Could you check a few things on this model? Use its own coordinates, in mm. Face numbers are marked on the shaded views. A direction names the side the tool comes from. Give positions to 0.01 mm unless a question says otherwise; leave off trailing zeros. Loops run counter-clockwise (first coordinate to the right, second up) from the corner with the lowest first, then second, coordinate; pieces in that order, holes last. Notation, with made-up numbers: M 57.5,-27.75 L 90.5,-27.75 A16 ccw 90.5,-5.75 Z; hole C 14.25,-24.5 d4. An arc over 180 degrees is marked long. Answer in a Markdown table with one row per item. Add a question column.
```python
from build123d import *

# Parameters (mm, degrees)
RESSALTO_EXTRUS_O1_DEPTH   = 15
CORTE_EXTRUS_O1_DEPTH      = 59.873508474
CORTE_EXTRUS_O1_DEPTH_BACK = 59.873508474
ESBO_O3_R                  = 5.5
CORTE_EXTRUS_O2_DEPTH      = 2
CORTE_EXTRUS_O2_DEPTH_BACK = 2
ESBO_O4_R                  = 11.5
ESBO_O6_R                  = 1.85
CORTE_EXTRUS_O4_DEPTH      = 64.251561246
CHANFRO1_SIZE              = 1.5


with BuildPart() as part:
    # Esboço1 → Ressalto-extrusão1 (new body)
    with BuildSketch(Plane(origin=(0, 0, 0), x_dir=(1, 0, 0), z_dir=(0, 1, 0))):
        with BuildLine():
            Line((3, 50), (3, 3))
            ThreePointArc((3, 3), (2.121320344, 0.878679656), (0, 0))
            Line((0, 0), (25.4, 0))
            ThreePointArc((25.4, 0), (23.278679656, 0.878679656), (22.4, 3))
            Line((22.4, 3), (22.4, 50))
            ThreePointArc((22.4, 50), (23.864466094, 53.535533906), (27.4, 55))
            Line((27.4, 55), (-2, 55))
            ThreePointArc((-2, 55), (1.535533906, 53.535533906), (3, 50))
        make_face()
    extrude(amount=RESSALTO_EXTRUS_O1_DEPTH)

    # Esboço3 → Corte-extrusão1 (cut, two sides: drawn at the far end of the back side and taken through both)
    with BuildSketch(Plane(origin=(12.7, 0, 0), x_dir=(0, 0, -1), z_dir=(1, 0, 0)).offset(-CORTE_EXTRUS_O1_DEPTH_BACK)):
        with Locations((26.5, 0)):
            Circle(ESBO_O3_R)
    extrude(amount=CORTE_EXTRUS_O1_DEPTH + CORTE_EXTRUS_O1_DEPTH_BACK, mode=Mode.SUBTRACT)

    # Esboço4 → Corte-extrusão2 (cut, two sides: drawn at the far end of the back side and taken through both)
    with BuildSketch(Plane(origin=(12.7, 0, 0), x_dir=(0, 0, -1), z_dir=(1, 0, 0)).offset(-CORTE_EXTRUS_O2_DEPTH_BACK)):
        with Locations((26.5, 0)):
            Circle(ESBO_O4_R)
    extrude(amount=CORTE_EXTRUS_O2_DEPTH + CORTE_EXTRUS_O2_DEPTH_BACK, mode=Mode.SUBTRACT)

    # Esboço6 → Corte-extrusão4 (cut, through all)
    with BuildSketch(Plane.XZ):
        with Locations(Location((16.4, -10.4, 0), (0, 0, 270))):
            Circle(ESBO_O6_R)
        with Locations(Location((9, -47, 0), (0, 0, 270))):
            Circle(ESBO_O6_R)
    extrude(amount=-CORTE_EXTRUS_O4_DEPTH, mode=Mode.SUBTRACT)

    # Chanfro1
    chanfro1_edges = [part.edges().sort_by_distance(p)[0] for p in [
        (16.4, 15, -8.55),
        (9, 15, -45.15),
    ]]
    chamfer(chanfro1_edges, length=CHANFRO1_SIZE)


solid = part.part
```
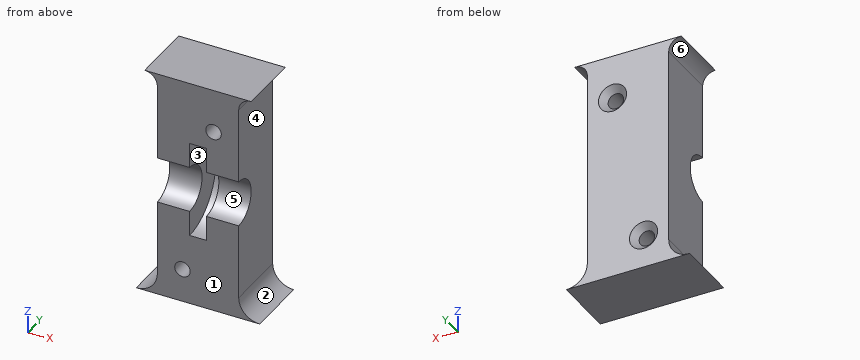
Item 1: If we mould it in two halves opening along X, with no side actions, what happens to the marked faces 1, 2 and 3? For each: +X half, -X half, draft (parallel to the pull), parting line (faces both ways), or undercut.
Item 2: For P1, Ø3.5, axis at y = 4.5, z = -26.5, coming from the -X side; P2, Ø3, axis at y = 4, z = -13, coming from the +X side, each with a flat end and sliding along its axis, tell me the tip position at first contact or that it passes through.
Item 3: Suppose I cut it at C-C (x = 16.4). List the corners of the cut face in (y, z) for me.
Item 4: Suppose I cut it at B-B (z = -10.4). List the corners of the cut face in (x, y) for me, then the cut area to 3 significant figures.
Item 5: Suppose I cut it at A-A (y = 4.5). List the corners of the cut face in (x, z) for me.
Item 6: Suppose I cut it at D-D (y = 12.5). List the corners of the cut face in (x, z) for me, then the cut area to 3 significant figures.
Item 7: For the marked faces 4, 5 and 6, which set-ups out of +Z, -Z, +X, -X, +Y, -Y let a thin tool reach every point of the face, with its end or its side?
Item 8: I need wall thicknesses on L1, parallel to X at y = 9.75, z = -31; L2, parallel to X at y = 10, z = -10.4; L3, parallel to Y at x = 8, z = -26.5. Which ranges of each line are inside material? Lowest first, please.
Values found:
| question | item | result |
|---|---|---|
| 1 | face 1 | draft |
| 1 | face 2 | +X half |
| 1 | face 3 | undercut |
| 2 | P1 | x = 3 |
| 2 | P2 | x = 22.4 |
| 3 | outline | M 0,-55 L 15,-55 L 15,-13.75 L 13.5,-12.25 L 0,-12.25 L 0,-21 A5.5 cw 0,-32 Z; M 0,-8.55 L 13.5,-8.55 L 15,-7.05 L 15,0 L 0,0 Z |
| 4 | outline | M 3,0 L 14.55,0 L 14.55,13.5 L 13.05,15 L 3,15 Z; M 18.25,0 L 22.4,0 L 22.4,15 L 19.75,15 L 18.25,13.5 Z |
| 4 | area | 233 mm² |
| 5 | outline | M -2,-55 L 27.4,-55 A5 cw 22.4,-50 L 22.4,-29.66 L 14.7,-29.66 L 14.7,-37.08 L 10.7,-37.08 L 10.7,-29.66 L 3,-29.66 L 3,-50 A5 cw Z; M 0,0 A3 cw 3,-3 L 3,-23.34 L 10.7,-23.34 L 10.7,-15.92 L 14.7,-15.92 L 14.7,-23.34 L 22.4,-23.34 L 22.4,-3 A3 cw 25.4,0 Z; hole C 9,-47 d3.7; hole C 16.4,-10.4 d3.7 |
| 6 | outline | M -2,-55 L 27.4,-55 A5 cw 22.4,-50 L 22.4,-3 A3 cw 25.4,0 L 0,0 A3 cw 3,-3 L 3,-50 A5 cw Z; hole C 9,-47 d3.7; hole C 16.4,-10.4 d3.7 |
| 6 | area | 1,060 mm² |
| 7 | face 4 | +X, +Y, -Y |
| 7 | face 5 | +X, -X, -Y |
| 7 | face 6 | -X, +Y, -Y |
| 8 | L1 | 3 to 10.7, 14.7 to 22.4 |
| 8 | L2 | 3 to 14.55, 18.25 to 22.4 |
| 8 | L3 | 5.5 to 15 |
